Read the model definition and answer for the solid it produces. Units are mm, in the model's axes. A direction names the side the tool comes from. Coordinates: 2 decimals unless noted, no trailing zeros. Write each loop counter-clockwise with the first axis right and the second up, starting at its lowest first coordinate (ties: lowest second). Pieces come first, ordered by that corner, then holes. Notation, with made-up numbers: M 80.5,78.5 L 94.5,78.5 A5 ccw 94.5,84.5 Z; hole C -8,-10 d7. An arc over 180 degrees is marked long. Use a Markdown table: item, result. Add a question column.
from build123d import *

# Parameters (mm, degrees)
F0_R     = 14.5
F1_DEPTH = 3.5
F2_R     = 9.7
F3_DEPTH = 16.1
F4_R     = 5.35
F5_DEPTH = 25.4
F6_R     = 1.016


with BuildPart() as f1:
    # F0 (on Right) → F1 (new body)
    with BuildSketch(Plane.YZ):
        Circle(F0_R)
    extrude(amount=F1_DEPTH)

    # F2 (on Right) → F3 (join)
    with BuildSketch(Plane.YZ):
        Circle(F2_R)
    extrude(amount=F3_DEPTH)

    # F4 (on Right) → F5 (cut)
    with BuildSketch(Plane.YZ):
        Circle(F4_R)
    extrude(amount=F5_DEPTH, mode=Mode.SUBTRACT)

    # F6
    f6_edges = [f1.edges().sort_by_distance(p)[0] for p in [
        (16.1, -9.7, 0),
    ]]
    fillet(f6_edges, radius=F6_R)


solid = f1.part
Item 1: Find section C-C on x = 9.75. Give the vertices of the cut face in (y, z), then the cut area to 3 significant figures.
Item 2: For faces 1 (the cylindrical face through (9.211, 9.252, 2.914)), 2 (the flat face through (0, 6, 0)), determine the directions among +Z, -Z, +X, -X, +Y, -Y from which every point of the face is accessible in a straight line to the end or side of a thin tool.
Item 3: Determine the mould class of faces 3 (the flat face through (16.1, 4, 4)), 4 (the cylindrical face through (7.937, -1.16, -5.223)), 5 (the cylindrical face through (1.726, 6.691, -12.864)) for opening direction Y: pulls with the +Y half, pulls with the -Y half, needs draft (parallel to the pull), parting line crosses it, or undercut.
Item 4: Find section A-A on y = 0. Give the vertices of the cut face in (x, z).
Item 5: Each of these flat-tipped pins is pushed along its axis until it touches: pin 1 (5 mm diameter, centred on y = -10.5, z = 3.5, fed in from -X); pin 2 (4 mm diameter, centred on x = 10, y = 9, fed in from -Z); pin 3 (8 mm diameter, centred on x = 5, z = 4.5, fed in from -Y); pin 4 (1 mm diameter, centred on y = 2.5, z = -11.5, fed in from +X). Where does it stop, or does it pass through?
Item 6: Consider probe 1 along Y at (x, z) = (5.25, 0); probe 2 along Y at (x, z) = (3.25, 0.25). Determine where each line is inside the solid, lowest interval first.
Item 7: Find section D-D on y = -11.25. Give the vertices of the cut face in (x, z), then the cut area to 3 significant figures.
Geometry says:
| question | item | result |
|---|---|---|
| 1 | outline | C 0,0 d19.4; hole C 0,0 d10.7 |
| 1 | area | 206 mm2 |
| 2 | face 1 | +X |
| 2 | face 2 | +Z, -Z, -X, +Y, -Y |
| 3 | face 3 | needs draft |
| 3 | face 4 | undercut |
| 3 | face 5 | parting line crosses it |
| 4 | outline | M 0,-14.5 L 3.5,-14.5 L 3.5,-9.7 L 15.08,-9.7 A1.02 ccw 16.1,-8.68 L 16.1,-5.35 L 0,-5.35 Z; M 0,5.35 L 16.1,5.35 L 16.1,8.68 A1.02 ccw 15.08,9.7 L 3.5,9.7 L 3.5,14.5 L 0,14.5 Z |
| 5 | pin 1 | stops at x = 0 |
| 5 | pin 2 | stops at z = -6.71 |
| 5 | pin 3 | stops at y = -14.48 |
| 5 | pin 4 | stops at x = 3.5 |
| 6 | probe 1 | y = -9.7 to -5.35, 5.35 to 9.7 |
| 6 | probe 2 | y = -14.5 to -5.34, 5.34 to 14.5 |
| 7 | outline | M 0,-9.15 L 3.5,-9.15 L 3.5,9.15 L 0,9.15 Z |
| 7 | area | 64.0 mm2 |
